The drawing under review shows one solid part. Ordinate dimensions are in mm from its lowest x, y, z. A direction names the side the tool comes from. Give positions to 0.01 mm unless a question says otherwise; leave off trailing zeros. Write each loop counter-clockwise with the first axis right and the second up, starting at its lowest first coordinate (ties: lowest second). Pieces come first, ordered by that corner, then holes. Notation, with made-up numbers: (55, 81) -> (82, 81) arc R15 cw to (82, 101) -> close; hole circle Ø10 at (6, 24.25). An arc over 180 degrees is marked (long way). Answer as a JSON object with one key per item and string values.
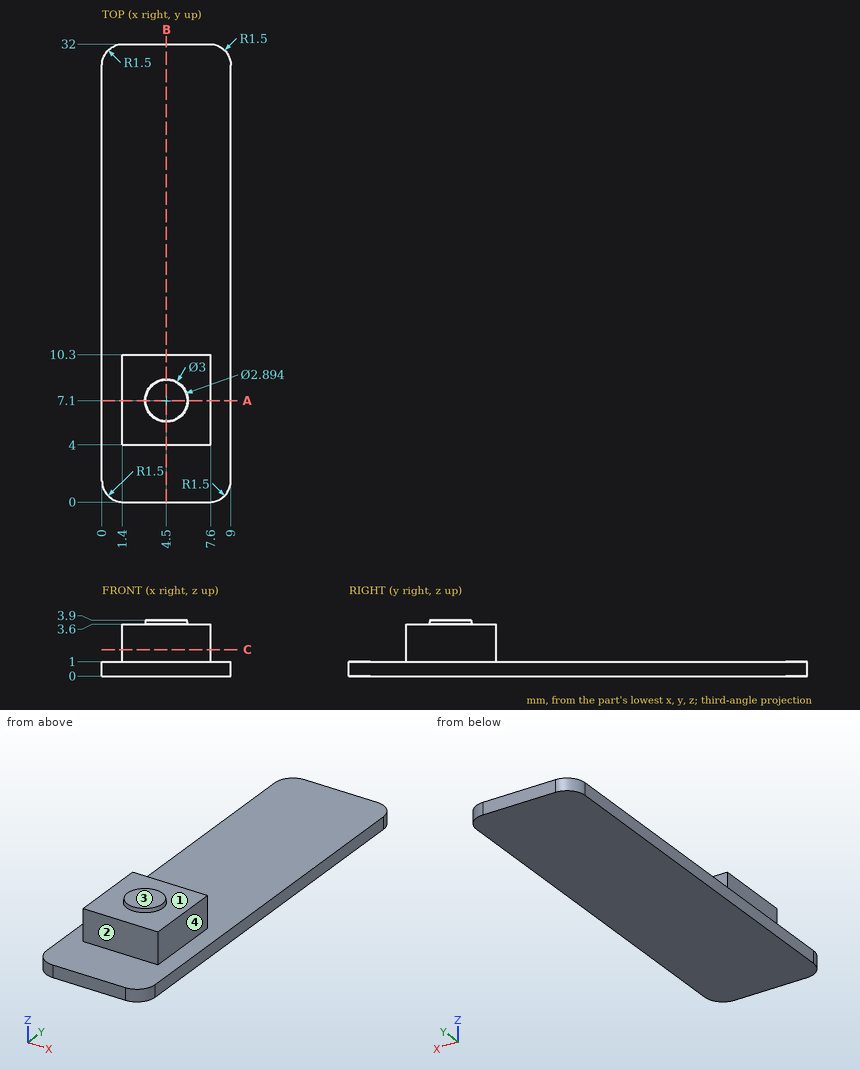
(1) For line 1 along Y through (x, z) = (6.25, 1.4); line 2 along Z through (x, y) = (1.25, 12); line 3 along Z through (x, y) = (1.5, 6.5), list the stretches that pass through material, from the lowest coordinate up.
Here are the results:
{"line 1": "y = 4 to 10.3", "line 2": "z = 0 to 1", "line 3": "z = 0 to 3.6"}
(2) We need section B-B, the plane x = 4.5. State the section outline as (y, z) points.
Here are the results:
{"outline": "(0, 0) -> (32, 0) -> (32, 1) -> (10.3, 1) -> (10.3, 3.6) -> (8.6, 3.6) -> (8.55, 3.9) -> (5.65, 3.9) -> (5.6, 3.6) -> (4, 3.6) -> (4, 1) -> (0, 1) -> close"}
(3) We need section C-C, the plane z = 1.85. State the section outline as (x, y) points.
Here are the results:
{"outline": "(1.4, 4) -> (7.6, 4) -> (7.6, 10.3) -> (1.4, 10.3) -> close"}
(4) Clearance check with flat-ended pins moving along their axes: pin 1 (2.5 mm diameter, centred on x = 3, y = 18.5, fed in from +Z); pin 2 (1 mm diameter, centred on x = 1.5, z = 3, fed in from +Y); pin 3 (2 mm diameter, centred on y = 5.5, z = 3, fed in from +X). State where each tip first meets the part, or that it passes through.
Here are the results:
{"pin 1": "stops at z = 1", "pin 2": "stops at y = 10.3", "pin 3": "stops at x = 7.6"}
(5) We need section A-A, the plane y = 7.1. State the section outline as (x, z) points, then the cut area to 3 significant figures.
Here are the results:
{"outline": "(0, 0) -> (9, 0) -> (9, 1) -> (7.6, 1) -> (7.6, 3.6) -> (6, 3.6) -> (5.95, 3.9) -> (3.05, 3.9) -> (3, 3.6) -> (1.4, 3.6) -> (1.4, 1) -> (0, 1) -> close", "area": "26.0 mm²"}
(6) For the marked faces 1, 2, 3 and 4, list the 3-axis set-ups (+Z, -Z, +X, -X, +Y, -Y) from which the entire face can be reached by the end or side of a thin tool; tool diameter is ignored.
Here are the results:
{"face 1": "+Z", "face 2": "+Z, +X, -X, -Y", "face 3": "+Z, +X, -X, +Y, -Y", "face 4": "+Z, +X, +Y, -Y"}
